The figure shows three views and two pictorial views of one solid part (mm, origin at its lowest corner). Answer the questions. Round coordinates to 2 decimals unless told otherwise and drop trailing zeros. Order: outer loops, then holes, each group sorted by start corner. A loop starts at its lowest first (then second) coordinate and runs counter-clockwise, first axis right, second up. Notation, with made-up numbers: (-34, 20) -> (18, 20) arc R23 ccw to (18, 53) -> close; hole circle Ø4 at (86.25, 68.5). An arc over 180 degrees is marked (long way). One line per item, written item: value. Start each with the question number.
1. Section C-C (y = 0.75) is taken. State how many separate pieces and enclosed holes the cut face has, then the cut area to 3 significant figures.
2. Section A-A (z = 75) is taken. Give the vertices of the cut face in (x, y), then the cut area to 3 significant figures.
3. Section D-D (z = 21) is taken. Give the vertices of the cut face in (x, y).
4. A flat-ended cylindrical pin translates along its axis: pin 1 Ø1.5 at (x, z) = (70.18, 21) entering from -Y. Find the tip coordinate at first contact, or state that the pin passes through.
5. Section B-B (x = 24.5) is taken. Give the vertices of the cut face in (y, z).
6. Consider line 1 (Z direction, x = 39, y = 1.4); line 2 (Z direction, x = 70, y = 1.8); line 3 (X direction, y = 1.7, z = 26.5). Determine where each line is inside the solid, lowest interval first.
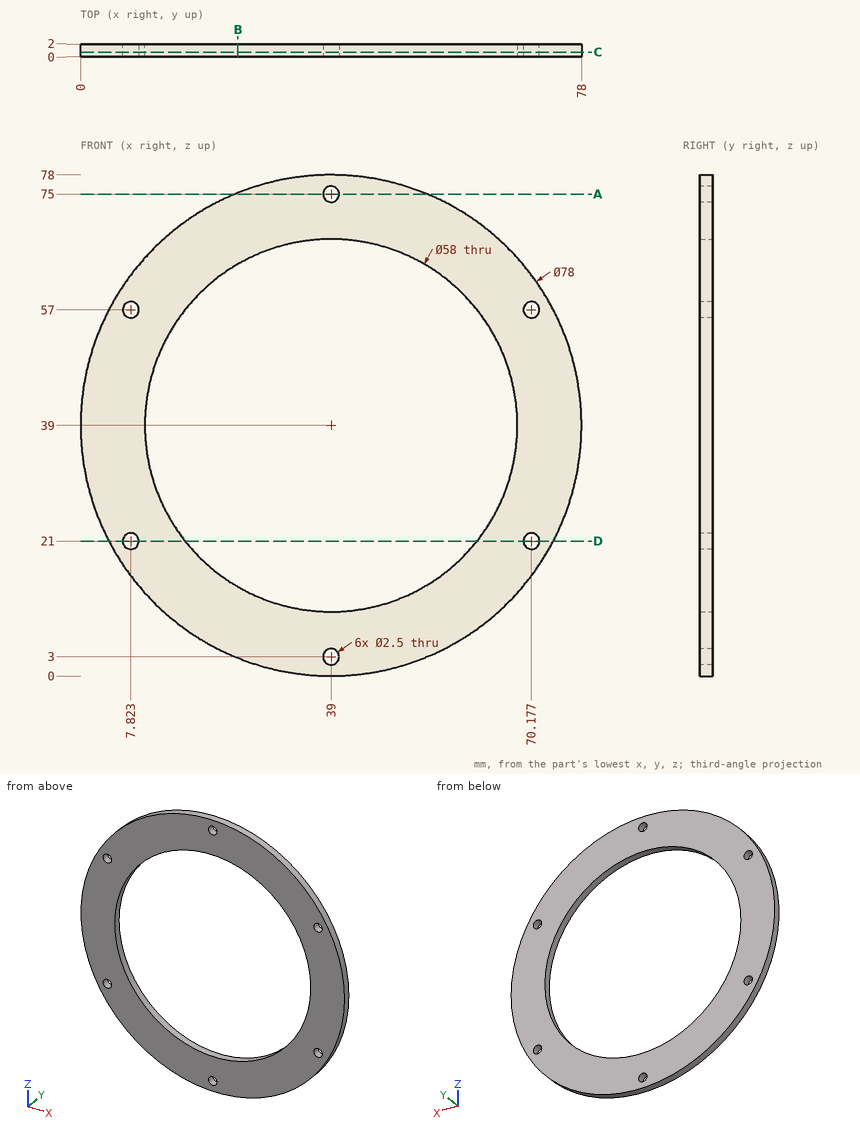
Answer:
1. separate pieces: 1
1. enclosed holes: 7
1. area: 2,110 mm^2
2. outline: (24, 0) -> (37.75, 0) -> (37.75, 2) -> (24, 2) -> close; (40.25, 0) -> (54, 0) -> (54, 2) -> (40.25, 2) -> close
2. area: 55.0 mm^2
3. outline: (4.4, 0) -> (6.57, 0) -> (6.57, 2) -> (4.4, 2) -> close; (9.07, 0) -> (16.26, 0) -> (16.26, 2) -> (9.07, 2) -> close; (61.74, 0) -> (68.93, 0) -> (68.93, 2) -> (61.74, 2) -> close; (71.43, 0) -> (73.6, 0) -> (73.6, 2) -> (71.43, 2) -> close
4. pin 1: through
5. outline: (0, 2.8) -> (2, 2.8) -> (2, 13.89) -> (0, 13.89) -> close; (0, 64.11) -> (2, 64.11) -> (2, 75.2) -> (0, 75.2) -> close
6. line 1: 0 to 1.75, 4.25 to 10, 68 to 73.75, 76.25 to 78
6. line 2: 15.34 to 19.76, 22.24 to 55.76, 58.24 to 62.66
6. line 3: 2.06 to 12.83, 65.17 to 75.94
